from build123d import *

# Parameters (mm, degrees)
F1_DEPTH = 5
F0_R     = 3.20253673
F0_R_2   = 2
F2_DEPTH = 2
F3_SCALE = 0.65


with BuildPart() as f1:
    # F0 (on Front) → F1 (new body)
    with BuildSketch(Plane.XZ):
        with BuildLine():
            ThreePointArc((11.8780601229, 6.1050535555), (12.3216651376, 6.5117042248), (12.4515672404, 7.0993058071))
            ThreePointArc((12.4515672404, 7.0993058071), (-2.0690604399, 18.3275702755), (-12.1281641394, 2.9738416091))
            ThreePointArc((-12.1281641394, 2.9738416091), (-9.0972996334, 1.1534404594), (-7.2768984837, 4.1843049654))
            ThreePointArc((-7.2768984837, 4.1843049654), (-0.7521606693, 13.4621883069), (7.4928698579, 5.6730423685))
            ThreePointArc((7.4928698579, 5.6730423685), (7.9363593577, 4.797971444), (8.914537434, 4.7231402306))
            Line((8.914537434, 4.7231402306), (11.8780601229, 6.1050535555))
        make_face()
    extrude(amount=F1_DEPTH)



with BuildPart() as f1b:
    # F0 (on Front) → F1, piece 2 (new body)
    with BuildSketch(Plane.XZ):
        with BuildLine():
            Line((1.75, -5.5069764979), (1.75, 6))
            ThreePointArc((1.75, 6), (0, 7.75), (-1.75, 6))
            Line((-1.75, 6), (-1.75, 0.8516268172))
            Line((-1.75, 0.8516268172), (-6.1623816362, 0.8516268172))
            ThreePointArc((-6.1623816362, 0.8516268172), (-7.9123816362, -0.8983731828), (-6.1623816362, -2.6483731828))
            Line((-6.1623816362, -2.6483731828), (-1.75, -2.6483731828))
            Line((-1.75, -2.6483731828), (-1.75, -3.7569764979))
            Line((-1.75, -3.7569764979), (-6.3856970519, -3.7569764979))
            ThreePointArc((-6.3856970519, -3.7569764979), (-7.3053342322, -4.0180952211), (-7.9505319996, -4.7235279761))
            Line((-7.9505319996, -4.7235279761), (-10.669789277, -10.1548852399))
            Line((-10.669789277, -10.1548852399), (-12.0862811892, -9.7137152259))
            ThreePointArc((-12.0862811892, -9.7137152259), (-14.2775052272, -10.8641661007), (-13.1270543524, -13.0553901387))
            Line((-13.1270543524, -13.0553901387), (-11.2260873483, -13.6474511541))
            ThreePointArc((-11.2260873483, -13.6474511541), (-10.0204395919, -13.5868674423), (-9.140865819, -12.7600622194))
            Line((-9.140865819, -12.7600622194), (-6.3856970519, -7.2569764979))
            Line((-6.3856970519, -7.2569764979), (0, -7.2569764979))
            ThreePointArc((0, -7.2569764979), (1.2374368671, -6.744413365), (1.75, -5.5069764979))
        make_face()
    extrude(amount=F1_DEPTH)


with BuildPart() as f1c:
    # F0 (on Front) → F1, piece 3 (new body)
    with BuildSketch(Plane.XZ):
        with Locations((0, -11.4851715043)):
            Circle(F0_R)
    extrude(amount=F1_DEPTH)


with BuildPart() as f1_1:
    add(f1.part)

    add(f1b.part)  # F2 merges F1b

    add(f1c.part)  # F2 merges F1c
    # F0 (on Front) → F2 (join)
    with BuildSketch(Plane.XZ):
        with BuildLine():
            ThreePointArc((3.7704463979, 19.6413781075), (0, 23.7874629637), (-3.7704463979, 19.6413781075))
            ThreePointArc((-3.7704463979, 19.6413781075), (0, -20), (3.7704463979, 19.6413781075))
        make_face()
        with Locations((0, -11.4851715043)):
            Circle(F0_R, mode=Mode.SUBTRACT)
        with BuildLine():
            ThreePointArc((-1.75, 6), (0, 7.75), (1.75, 6))
            Line((1.75, 6), (1.75, -5.5069764979))
            ThreePointArc((1.75, -5.5069764979), (1.2374368671, -6.744413365), (0, -7.2569764979))
            Line((0, -7.2569764979), (-6.3856970519, -7.2569764979))
            Line((-6.3856970519, -7.2569764979), (-9.140865819, -12.7600622194))
            ThreePointArc((-9.140865819, -12.7600622194), (-10.0204395919, -13.5868674423), (-11.2260873483, -13.6474511541))
            Line((-11.2260873483, -13.6474511541), (-13.1270543524, -13.0553901387))
            ThreePointArc((-13.1270543524, -13.0553901387), (-14.2775052272, -10.8641661007), (-12.0862811892, -9.7137152259))
            Line((-12.0862811892, -9.7137152259), (-10.669789277, -10.1548852399))
            Line((-10.669789277, -10.1548852399), (-7.9505319996, -4.7235279761))
            ThreePointArc((-7.9505319996, -4.7235279761), (-7.3053342322, -4.0180952211), (-6.3856970519, -3.7569764979))
            Line((-6.3856970519, -3.7569764979), (-1.75, -3.7569764979))
            Line((-1.75, -3.7569764979), (-1.75, -2.6483731828))
            Line((-1.75, -2.6483731828), (-6.1623816362, -2.6483731828))
            ThreePointArc((-6.1623816362, -2.6483731828), (-7.9123816362, -0.8983731828), (-6.1623816362, 0.8516268172))
            Line((-6.1623816362, 0.8516268172), (-1.75, 0.8516268172))
            Line((-1.75, 0.8516268172), (-1.75, 6))
        make_face(mode=Mode.SUBTRACT)
        with BuildLine():
            ThreePointArc((-12.1281641394, 2.9738416091), (-2.0690604399, 18.3275702755), (12.4515672404, 7.0993058071))
            ThreePointArc((12.4515672404, 7.0993058071), (12.3216651376, 6.5117042248), (11.8780601229, 6.1050535555))
            Line((11.8780601229, 6.1050535555), (8.914537434, 4.7231402306))
            ThreePointArc((8.914537434, 4.7231402306), (7.9363593577, 4.797971444), (7.4928698579, 5.6730423685))
            ThreePointArc((7.4928698579, 5.6730423685), (-0.7521606693, 13.4621883069), (-7.2768984837, 4.1843049654))
            ThreePointArc((-7.2768984837, 4.1843049654), (-9.0972996334, 1.1534404594), (-12.1281641394, 2.9738416091))
        make_face(mode=Mode.SUBTRACT)
        with Locations((0, 20.6641051918)):
            Circle(F0_R_2, mode=Mode.SUBTRACT)
    extrude(amount=F2_DEPTH)


with BuildPart() as f1_2:
    # F3: moved
    add(f1_1.part.scale(F3_SCALE).moved(Location((0, 0, 0))))


solid = f1_2.part
Can you work these out from the model? Positions are in its coordinate system, mm. A direction names the side the tool comes from. Give positions to 0.01 mm unless a question says otherwise; leave off trailing zeros. Order: outer loops, then holes, each group sorted by start corner. A loop starts at its lowest first (then second) coordinate and runs counter-clockwise, first axis right, second up. Notation, with made-up numbers: M -13,88 L 21,88 A24 ccw 21,101 Z; hole C -17.5,4 d1. An arc over 180 degrees is marked long. Use one line per item in the form item = value. Start each with the question number.
Item 1: If we section it at C-C (z = 9.25): Write out the boundary of the cut face in (x, y) (3 decimals).
Item 2: If we section it at D-D (z = 0): Write out the boundary of the cut face in (x, y).
Item 3: We'd pull the mould along X, two halves only. Please class faces 4 (the cylindrical face through (0.8, -2.26, -4.39)), 5 (the cylindrical face through (5.151, -2.261, 3.124)), 6 (the flat face through (-3, -3.25, -1)): +X half, -X half, draft (parallel to the pull), parting line (faces both ways), or undercut.
Item 4: If we section it at B-B (x = -6.5): Write out the boundary of the cut face in (y, z) (3 decimals), then the cut area to 3 significant figures.
Item 5: For faces 1 (the cylindrical face through (0.025, -2.261, 5.037)), 2 (the cylindrical face through (-5.143, -2.261, -0.559)), 3 (the flat face through (6.74, -2.26, 3.51)), which set-ups out of +Z, -Z, +X, -X, +Y, -Y let a thin tool reach every point of the face, with its end or its side?
Item 6: Will these pins go through, and if not, where does the flat tip stop? pin 1 Ø1 at (x, y) = (-2.5, -2) entering from +Z (3 decimals); pin 2 Ø1 at (x, y) = (-2, -2.5) entering from -Z; pin 3 Ø1 at (x, y) = (-3, -2.5) entering from -Z.
Item 7: If we section it at A-A (y = -1.7): State how many separate pieces and enclosed holes the cut face has, then the cut area to 3 significant figures.
Item 8: If I drill on line 1 along Z through (x, y) = (-0.75, -1.4); line 2 along Z through (x, y) = (0, -0.9); line 3 along Y through (x, z) = (-9.5, 2), over which ranges is the centre line in solid material (lowest first)?
Outcome:
q1.outline = M -9.134,-1.3 L -6.115,-1.3 L -6.115,-3.25 L 6.115,-3.25 L 6.115,-1.3 L 9.134,-1.3 L 9.134,0 L -9.134,0 Z
q2.outline = M -13,-1.3 L -4.98,-1.3 L -4.98,-3.25 L 1.14,-3.25 L 1.14,-1.3 L 13,-1.3 L 13,0 L -13,0 Z
q3.face_4 = +X half
q3.face_5 = undercut
q3.face_6 = draft
q4.outline = M -3.25,-8.826 L -1.3,-8.826 L -1.3,-11.258 L 0,-11.258 L 0,11.258 L -1.3,11.258 L -1.3,8.775 L -3.25,8.775 L -3.25,0.713 L -1.3,0.713 L -1.3,-5.731 L -3.25,-5.731 Z
q4.area = 51.0 mm2
q5.face_1 = -Y
q5.face_2 = -X, -Y
q5.face_3 = -Z, +X, -Y
q6.pin_1 = 11.775
q6.pin_2 = -8.91
q6.pin_3 = -4.72
q7.separate_pieces = 3
q7.enclosed_holes = 0
q7.area = 142 mm2
q8.line_1 = -9.41 to -5.52, -4.72 to 4.76, 8.72 to 11.99
q8.line_2 = -13 to 12.13, 14.73 to 15.46
q8.line_3 = -1.3 to 0
